```python
from build123d import *

# Parameters (mm, degrees)
SKETCH1_R               = 6.477
BOSS_EXTRUDE1_DEPTH     = 12.7
SKETCH2_W               = 4.064
SKETCH2_H               = 58.166
CUT_EXTRUDE1_DEPTH      = 2.032
CUT_EXTRUDE1_DRAFT      = -15
SKETCH3_W               = 4.064
SKETCH3_H               = 58.166
CUT_EXTRUDE2_DEPTH      = 2.032
CUT_EXTRUDE2_DRAFT      = -15
CUT_EXTRUDE3_DEPTH      = 113.937209103
CUT_EXTRUDE3_DEPTH_BACK = 10.16
SKETCH4_OUTSIDE_W       = 47.17
SKETCH4_OUTSIDE_H       = 39.55
SKETCH4_OUTSIDE_R       = 10.16


with BuildPart() as part:
    # Sketch1 → Boss-Extrude1 (new body)
    with BuildSketch(Plane.XY):
        with BuildLine():
            Line((-10.16, 0), (-10.16, 12.7))
            Line((-10.16, 12.7), (-3.302, 28.175956627))
            Line((-3.302, 28.175956627), (-3.302, 91.991545598))
            ThreePointArc((-3.302, 91.991545598), (0, 111.76), (3.302, 91.991545598))
            Line((3.302, 91.991545598), (3.302, 28.175956627))
            Line((3.302, 28.175956627), (10.16, 12.7))
            Line((10.16, 12.7), (10.16, 0))
            ThreePointArc((10.16, 0), (0, -10.16), (-10.16, 0))
        make_face()
        with Locations(Location((0, 0, 0), (0, 0, 180))):
            Circle(SKETCH1_R, mode=Mode.SUBTRACT)
        with Locations(Location((0, 101.6, 0), (0, 0, 180))):
            Circle(SKETCH1_R, mode=Mode.SUBTRACT)
    extrude(amount=BOSS_EXTRUDE1_DEPTH)


with BuildPart() as cut_extrude1_tool:
    # Sketch2 → Cut-Extrude1 (with draft: the straight prism first)
    with BuildSketch(Plane.XY.offset(12.7)):
        with Locations((0, 60.325)):
            Rectangle(SKETCH2_W, SKETCH2_H)
    extrude(amount=-CUT_EXTRUDE1_DEPTH)
    # Cut-Extrude1: the draft: its side faces are tilted about the plane it starts from
    cut_extrude1_sides = [cut_extrude1_tool.faces().sort_by_distance(p)[0] for p in [
        (-2.032, 60.325, 11.684),
        (0, 31.242, 11.684),
        (2.032, 60.325, 11.684),
        (0, 89.408, 11.684),
    ]]
    draft(cut_extrude1_sides, Plane.XY.offset(12.7), CUT_EXTRUDE1_DRAFT)


with BuildPart() as part_1:
    add(part.part)

    # Cut-Extrude1: cut by cut_extrude1_tool
    add(cut_extrude1_tool.part, mode=Mode.SUBTRACT)


with BuildPart() as cut_extrude2_tool:
    # Sketch3 → Cut-Extrude2 (with draft: the straight prism first)
    with BuildSketch(Plane(origin=(0, 0, 0), x_dir=(-1, 0, 0), z_dir=(0, 0, -1))):
        with Locations((0, 60.325)):
            Rectangle(SKETCH3_W, SKETCH3_H)
    extrude(amount=-CUT_EXTRUDE2_DEPTH)
    # Cut-Extrude2: the draft: its side faces are tilted about the plane it starts from
    cut_extrude2_sides = [cut_extrude2_tool.faces().sort_by_distance(p)[0] for p in [
        (2.032, 60.325, 1.016),
        (0, 31.242, 1.016),
        (-2.032, 60.325, 1.016),
        (0, 89.408, 1.016),
    ]]
    draft(cut_extrude2_sides, Plane(origin=(0, 0, 0), x_dir=(-1, 0, 0), z_dir=(0, 0, -1)), CUT_EXTRUDE2_DRAFT)


with BuildPart() as part_2:
    add(part_1.part)

    # Cut-Extrude2: cut by cut_extrude2_tool
    add(cut_extrude2_tool.part, mode=Mode.SUBTRACT)

    # Sketch4 outside → Cut-Extrude3 (cut, two sides: drawn at the far end of the back side and taken through both)
    with BuildSketch(Plane(origin=(0, 0, 0), x_dir=(1, 0, 0), z_dir=(0, 1, 0)).offset(-CUT_EXTRUDE3_DEPTH_BACK)):
        with Locations((0, -6.35)):
            Rectangle(SKETCH4_OUTSIDE_W, SKETCH4_OUTSIDE_H)
        with Locations((0, -6.35)):
            Circle(SKETCH4_OUTSIDE_R, mode=Mode.SUBTRACT)
    extrude(amount=CUT_EXTRUDE3_DEPTH + CUT_EXTRUDE3_DEPTH_BACK, mode=Mode.SUBTRACT)


solid = part_2.part
```
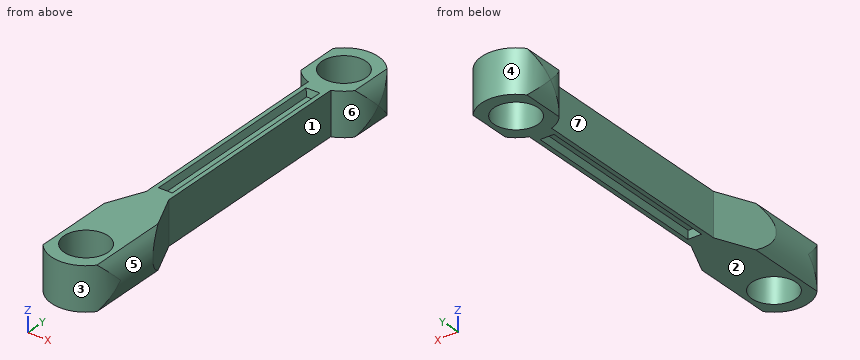
Model file for the job. Use its own axes, mm. Face numbers are marked on the shaded views. A direction names the side the tool comes from. Coordinates: 2 decimals unless noted, no trailing zeros. Order: outer loops, then holes, each group sorted by start corner. A loop starts at its lowest first (then second) coordinate and runs counter-clockwise, first axis right, second up. Notation, with made-up numbers: (4.5, -34.75) -> (45.5, -34.75) arc R16 ccw to (45.5, -14.75) -> close; hole circle Ø5 at (-25.5, -7). An arc over 180 degrees is marked (long way). Answer as a JSON object with one key per item and string values. Group by question number.
1) Cut at A-A, the plane x = 0. Write the cut outline in (y, z).
2) Cut at B-B, the plane y = 1. Write the cut outline in (x, z).
3) Flat gauge pins, fed straight in: pin 1 (1 mm diameter, centred on x = 7.5, z = 2, fed in from +Y); pin 2 (6 mm diameter, centred on x = 5.5, z = 6, fed in from -Y); pin 3 (1.5 mm diameter, centred on y = 30, z = 10, fed in from +X); pin 4 (3 mm diameter, centred on x = -6, y = 55, fed in from +Z). Where does each tip first touch, or does it go through?
4) Cut at C-C, the plane y = 59. Write the cut outline in (x, z), then the cut area to 3 significant figures.
5) Which spindle directions (+Z, -Z, +X, -X, +Y, -Y) get a long thin tool onto all of the face, cutting with end or side? Do the marked faces 5, 6 and 7. Say none if no direction does.
6) Pull direction Y, two halves, no side cores. Call the marked faces 1, 2, 3 and 4: +Y half, -Y half, draft (parallel to the pull), parting line (faces both ways), or undercut.
7) Cut at D-D, the plane z = 5.25. Write the cut outline in (x, y), then the cut area to 3 significant figures.
8) Drill centre lines: L1, parallel to Y at x = 5.75, z = 6.5; L2, parallel to Y at x = -3, z = 9.75; L3, parallel to Y at x = -2.75, z = 8.5. Where is each one in solid material? Low to high.
Check values:
{
 "1": {"outline": "(-10.16, 0) -> (-6.48, 0) -> (-6.48, 12.7) -> (-10.16, 12.7) -> close; (6.48, 0) -> (31.24, 0) -> (31.79, 2.03) -> (88.86, 2.03) -> (89.41, 0) -> (95.12, 0) -> (95.12, 12.7) -> (89.41, 12.7) -> (88.86, 10.67) -> (31.79, 10.67) -> (31.24, 12.7) -> (6.48, 12.7) -> close; (108.08, 0) -> (111.76, 0) -> (111.76, 12.7) -> (108.08, 12.7) -> close"},
 "2": {"outline": "(-7.93, 0) -> (-6.4, 0) -> (-6.4, 12.7) -> (-7.93, 12.7) arc R10.16 ccw to start; (6.4, 0) -> (7.93, 0) arc R10.16 ccw to (7.93, 12.7) -> (6.4, 12.7) -> close"},
 "3": {"pin 1": "stops at y = 108.96", "pin 2": "stops at y = -9.85", "pin 3": "stops at x = 3.3", "pin 4": "passes through"},
 "4": {"outline": "(-3.3, 0) -> (-2.03, 0) -> (-1.49, 2.03) -> (1.49, 2.03) -> (2.03, 0) -> (3.3, 0) -> (3.3, 12.7) -> (2.03, 12.7) -> (1.49, 10.67) -> (-1.49, 10.67) -> (-2.03, 12.7) -> (-3.3, 12.7) -> close", "area": "69.6 mm²"},
 "5": {"face 5": "+X, +Y, -Y", "face 6": "+Z, -Z, +X", "face 7": "+Z, -Z, -X"},
 "6": {"face 1": "undercut", "face 2": "draft", "face 3": "-Y half", "face 4": "undercut"},
 "7": {"outline": "(-10.1, -1.1) arc R10.16 ccw to (10.1, -1.1) -> (10.1, 12.83) -> (3.3, 28.18) -> (3.3, 91.99) arc R10.16 ccw to (10.1, 100.5) -> (10.1, 102.7) arc R10.16 ccw to (-10.1, 102.7) -> (-10.1, 100.5) arc R10.16 ccw to (-3.3, 91.99) -> (-3.3, 28.18) -> (-10.1, 12.83) -> close; hole circle Ø12.95 at (0, 0); hole circle Ø12.95 at (0, 101.6)", "area": "1,110 mm²"},
 "8": {"L1": "y = -8.38 to -2.98, 2.98 to 22.65, 93.22 to 98.62, 104.58 to 109.98", "L2": "y = -9.71 to -5.74, 5.74 to 95.86, 107.34 to 111.31", "L3": "y = -9.78 to -5.86, 5.86 to 95.74, 107.46 to 111.38"}
}
